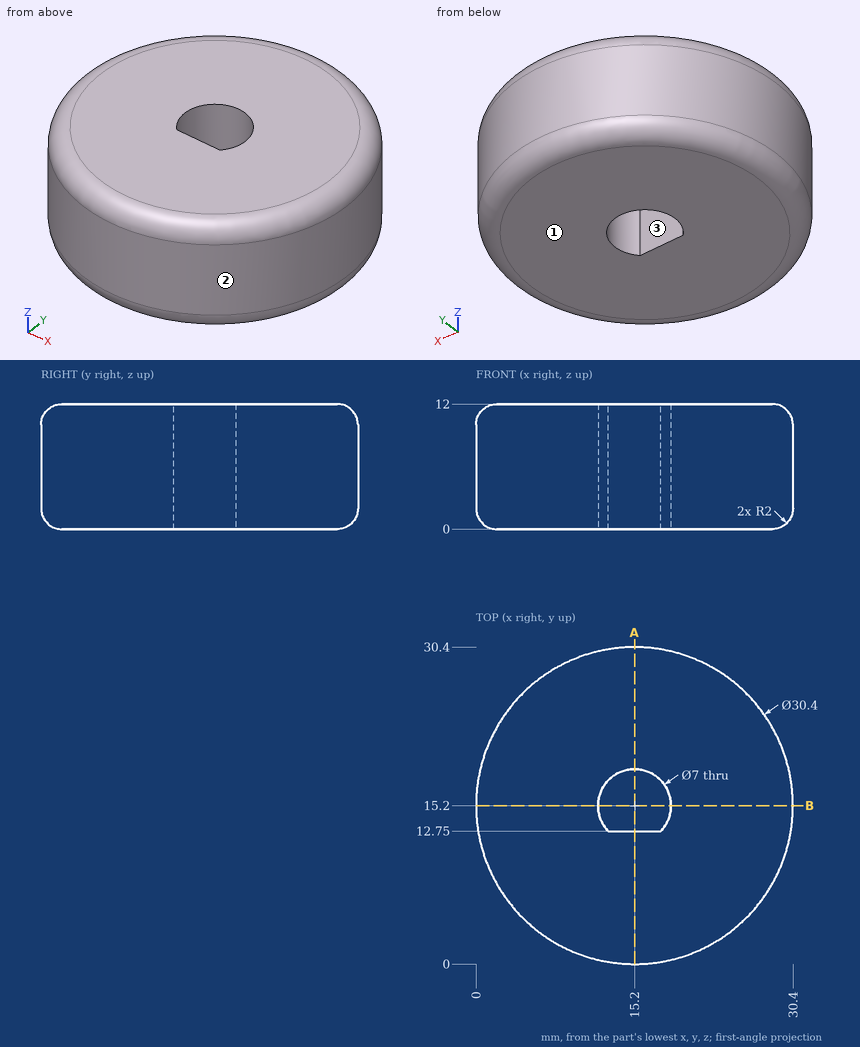
Input: dimensioned drawing with shaded views. Units: mm. Origin: part minimum x, y, z. Round coordinates to 2 decimals unless told otherwise and drop trailing zeros. Loops run counter-clockwise (first coordinate to the right, second up) from the corner with the lowest first, then second, coordinate; pieces in that order, holes last. Notation, with made-up numbers: M 60,28 L 111,28 A12 cw 111,41 Z; hole C -1.75,57.5 d3. An arc over 180 degrees is marked long. Return JSON: item names as keys, results as strings. Group by question number.
1. Section query B-B on y = 15.2. Output: boundary loops of the cut face in (x, z), and give its area (3 significant figures).
2. Mould query, pull axis X, two halves, no side actions, for the marked faces 1, 2 and 3. Classes: released by +X, released by -X, zero draft, split by the parting line, or undercut.
3. Section query A-A on x = 15.2. Output: boundary loops of the cut face in (y, z).
4. Material intervals for line 1 along Y through (x, z) = (15.2, 4.5); line 2 along Y through (x, z) = (14, 5.75); line 3 along Y through (x, z) = (28, 8) (1 decimal), sorted ascending. Write a range as from..to.
5. Pin query (flat end, axial travel): pin 1 (2 mm diameter, centred on y = 8, z = 9.5, fed in from +X); pin 2 (10 mm diameter, centred on x = 5.5, y = 17, fed in from -Z); pin 3 (1 mm diameter, centred on y = 4.5, z = 3.5, fed in from +X); pin 4 (1.5 mm diameter, centred on x = 25, z = 2, fed in from +Y). Return the tip coordinate at first contact, or that it passes through.
Checks:
{
 "1": {"outline": "M 0,2 A2 ccw 2,0 L 11.7,0 L 11.7,12 L 2,12 A2 ccw 0,10 Z; M 18.7,0 L 28.4,0 A2 ccw 30.4,2 L 30.4,10 A2 ccw 28.4,12 L 18.7,12 Z", "area": "277 mm²"},
 "2": {"face 1": "zero draft", "face 2": "split by the parting line", "face 3": "undercut"},
 "3": {"outline": "M 0,2 A2 ccw 2,0 L 12.75,0 L 12.75,12 L 2,12 A2 ccw 0,10 Z; M 18.7,0 L 28.4,0 A2 ccw 30.4,2 L 30.4,10 A2 ccw 28.4,12 L 18.7,12 Z"},
 "4": {"line 1": "y = 0..12.75, 18.7..30.4", "line 2": "y = 0.05..12.75, 18.49..30.35", "line 3": "y = 7..23.4"},
 "5": {"pin 1": "stops at x = 29.08", "pin 2": "stops at z = 0", "pin 3": "stops at x = 26.47", "pin 4": "stops at y = 27.41"}
}
